Input: part model. Units: mm. Frame: model coordinates. A direction names the side the tool comes from. Give positions to 0.01 mm unless a question says otherwise; leave off trailing zeros. Write each loop counter-clockwise with the first axis right and the second up, starting at its lowest first coordinate (ties: lowest second). Pieces come first, ordered by that corner, then holes. Notation, with made-up numbers: (60, 59) - (114, 59) arc R8 ccw to (114, 71) - close; hole circle Ø10 at (-32, 15.25). An arc over 180 degrees is marked (long way). Use a Markdown table: item, result. Add a question column.
1. Section query A-A, the plane z = 22.25. Return loops of the section in (x, y), plus the area to 3 significant figures.
2. Pin query (flat end, axial travel): pin 1 (12 mm diameter, centred on y = -2.5, z = 13, fed in from -X); pin 2 (4 mm diameter, centred on x = 5.5, y = 3.5, fed in from +Z); pin 3 (7 mm diameter, centred on y = -5.5, z = 22, fed in from -X). Return the tip coordinate at first contact, or that it passes through.
3. Section query D-D, the plane z = 6.5. Return loops of the section in (x, y).
4. Section query C-C, the plane x = -57.5. Return loops of the section in (y, z).
5. Section query B-B, the plane y = 42.5. Return loops of the section in (x, z), plus the area to 3 significant figures.
6. Material intervals for probe 1 along X at (y, z) = (21, 19.5); probe 2 along Z at (x, y) = (3.5, 47.5); probe 3 along X at (y, z) = (-8.5, 8.25), sorted ascending.
7. Mould query, pull axis X, two halves, no side actions, for faces 1 (the flat face through (45, 4, 25.4)), 2 (the flat face through (76.99, 3, 13)), 3 (the flat face through (7, 3, 19.132)). Classes: released by +X, released by -X, zero draft, split by the parting line, or undercut.
8. Set-up query: faces 4 (the flat face through (-3, 4, 0)), 5 (the flat face through (13.767, 3, 22)). Return all of +Z, -Z, +X, -X, +Y, -Y with unobstructed straight access to the full face (end or side cutting, diameter ignored); none if empty.
```python
from build123d import *

# Parameters (mm, degrees)
F0_W     = 156.9909751415
F0_H     = 101.4308109879
F1_DEPTH = 25.4
F3_DEPTH = 127.8210822493
F4_W     = 13.7669481337
F4_H     = 6.2678030968
F5_DEPTH = 157.0622399449


with BuildPart() as f1:
    # F0 (on Top) → F1 (new body)
    with BuildSketch(Plane.XY):
        with Locations((-1.5058219433, 3.2995529473)):
            Rectangle(F0_W, F0_H)
    extrude(amount=F1_DEPTH)

    # F2 (on face) → F3 (cut)
    with BuildSketch(Plane.XZ.offset(47.4158525467)):
        Polygon((-80.001309514, 25.4), (-80.001309514, 0), (-54.3336644769, 25.4), align=None)
    extrude(amount=-F3_DEPTH, mode=Mode.SUBTRACT)

    # F4 (on face) → F5 (cut)
    with BuildSketch(Plane.XZ.offset(47.4158525467)):
        with Locations((6.8834740669, 22.2660984516)):
            Rectangle(F4_W, F4_H)
    extrude(amount=-F5_DEPTH, mode=Mode.SUBTRACT)


solid = f1.part
```
Result sheet:
| question | item | result |
|---|---|---|
| 1 | outline | (-57.52, -47.42) - (0, -47.42) - (0, 54.01) - (-57.52, 54.01) - close; (13.77, -47.42) - (76.99, -47.42) - (76.99, 54.01) - (13.77, 54.01) - close |
| 1 | area | 12,200 mm² |
| 2 | pin 1 | stops at x = -72.93 |
| 2 | pin 2 | stops at z = 19.13 |
| 2 | pin 3 | stops at x = -61.31 |
| 3 | outline | (-73.43, -47.42) - (76.99, -47.42) - (76.99, 54.01) - (-73.43, 54.01) - close |
| 4 | outline | (-47.42, 0) - (54.01, 0) - (54.01, 22.27) - (-47.42, 22.27) - close |
| 5 | outline | (-80, 0) - (76.99, 0) - (76.99, 25.4) - (13.77, 25.4) - (13.77, 19.13) - (0, 19.13) - (0, 25.4) - (-54.33, 25.4) - close |
| 5 | area | 3,580 mm² |
| 6 | probe 1 | x = -60.3 to 0, 13.77 to 76.99 |
| 6 | probe 2 | z = 0 to 19.13 |
| 6 | probe 3 | x = -71.66 to 76.99 |
| 7 | face 1 | zero draft |
| 7 | face 2 | released by +X |
| 7 | face 3 | undercut |
| 8 | face 4 | -Z, +X, -X, +Y, -Y |
| 8 | face 5 | +Z, +Y, -Y |
